Answer from the drawing. Dimensions are ordinates in mm from the lowest x, y and z of the part. Coordinates: 2 decimals unless noted, no trailing zeros. Write each loop counter-clockwise with the first axis right and the second up, starting at its lowest first coordinate (ties: lowest second). Pieces come first, ordered by that corner, then holes.
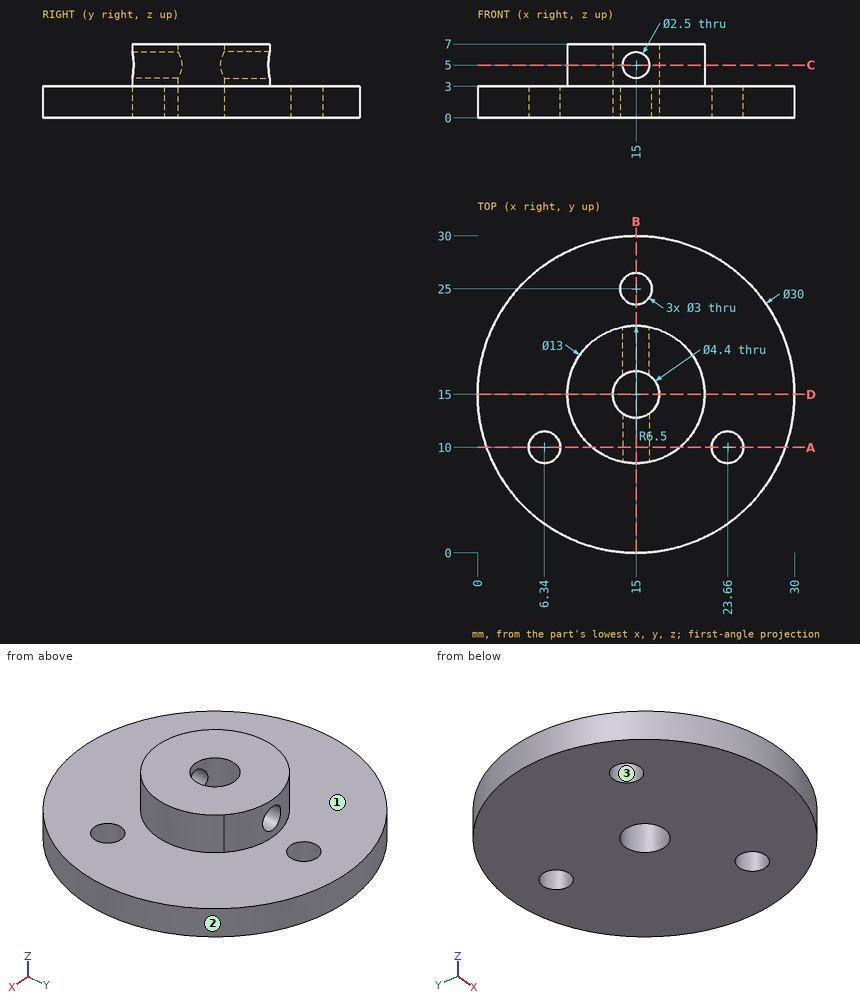
(1) Each of these flat-tipped pins is pushed along its axis until it touches: pin 1 (1.8 mm diameter, centred on x = 15, y = 25, fed in from +Z); pin 2 (1 mm diameter, centred on x = 11.5, z = 4, fed in from -Y); pin 3 (5 mm diameter, centred on x = 23.66, y = 10, fed in from +Z); pin 4 (3 mm diameter, centred on x = 15, z = 5, fed in from -Y). Where does it stop, or does it pass through?
(2) Find the intervals of material crossed by probe 1 along Y at (x, z) = (15, 1.75); probe 2 along X at (y, z) = (15, 5); probe 3 along X at (y, z) = (14.5, 5.5), in increasing order.
(3) Section A-A, the plane y = 10 is taken. Write down the section's boundary in (x, z).
(4) Section D-D, the plane y = 15 is taken. Write down the section's boundary in (x, z).
(5) For a pull along X with two mould halves and no side action, classify the marked faces 1, 2 and 3 as pulls with the +X half, pulls with the -X half, needs draft (parallel to the pull), parting line crosses it, or undercut.
(6) Section C-C, the plane z = 5 is taken. Write down the section's boundary in (x, y).
(7) Section B-B, the plane x = 15 is taken. Write down the section's boundary in (y, z).
Solution:
1. pin 1: passes through
1. pin 2: stops at y = 9.23
1. pin 3: stops at z = 3
1. pin 4: stops at y = 8.5
2. probe 1: y = 0 to 12.8, 17.2 to 23.5, 26.5 to 30
2. probe 2: x = 8.5 to 12.8, 17.2 to 21.5
2. probe 3: x = 8.52 to 12.86, 17.14 to 21.48
3. outline: (0.86, 0) - (4.84, 0) - (4.84, 3) - (0.86, 3) - close; (7.84, 0) - (22.16, 0) - (22.16, 3) - (19.15, 3) - (19.15, 7) - (10.85, 7) - (10.85, 3) - (7.84, 3) - close; (25.16, 0) - (29.14, 0) - (29.14, 3) - (25.16, 3) - close; hole circle Ø2.5 at (15, 5)
4. outline: (0, 0) - (12.8, 0) - (12.8, 7) - (8.5, 7) - (8.5, 3) - (0, 3) - close; (17.2, 0) - (30, 0) - (30, 3) - (21.5, 3) - (21.5, 7) - (17.2, 7) - close
5. face 1: needs draft
5. face 2: parting line crosses it
5. face 3: undercut
6. outline: (13.75, 8.62) - (13.75, 13.19) arc R2.2 cw to (13.75, 16.81) - (13.75, 21.38) arc R6.5 ccw to start; (16.25, 8.62) arc R6.5 ccw to (16.25, 21.38) - (16.25, 16.81) arc R2.2 cw to (16.25, 13.19) - close
7. outline: (0, 0) - (12.8, 0) - (12.8, 3.75) - (8.5, 3.75) - (8.5, 3) - (0, 3) - close; (8.5, 6.25) - (12.8, 6.25) - (12.8, 7) - (8.5, 7) - close; (17.2, 0) - (23.5, 0) - (23.5, 3) - (21.5, 3) - (21.5, 3.75) - (17.2, 3.75) - close; (17.2, 6.25) - (21.5, 6.25) - (21.5, 7) - (17.2, 7) - close; (26.5, 0) - (30, 0) - (30, 3) - (26.5, 3) - close
